Check sheet for the drawn part. Datum: minimum x, y, z corner. Units: mm. Give positions to 0.01 mm unless a question says otherwise; leave off trailing zeros. Order: outer loops, then holes, each group sorted by start corner. A loop starts at its lowest first (then second) coordinate and runs counter-clockwise, first axis right, second up. Notation, with made-up numbers: M 33.5,-34.5 L 64.5,-34.5 A34 cw 64.5,4.5 Z; hole C 55,84 d11. An arc over 180 degrees is marked long. Put each result on its own line as item: value. Start each with the question number.
Q1. Section check C-C on z = 6.5. Record the cut outline in (x, y), then the cut area to 3 significant figures.
Q2. Section check A-A on y = 13. Record the cut outline in (x, z), then the cut area to 3 significant figures.
Q3. Material ranges on L1, parallel to Y at x = 13, z = 4; L2, parallel to Y at x = 9, z = 7.25; L3, parallel to X at y = 10.5, z = 4.25, recorded low to high.
Q4. Mould release check, pull along Y, two halves, no side actions. Record for the marked faces 1, 2 and 3: +Y half, -Y half, draft (parallel to the pull), parting line (faces both ways), or undercut.
Q5. Go/stop test with flat-tipped pins: pin 1 (1 mm diameter, centred on x = 15.5, z = 4, fed in from -Y); pin 2 (2 mm diameter, centred on x = 9.5, z = 1.5, fed in from +Y); pin 3 (8 mm diameter, centred on x = 13, y = 13, fed in from -Z); pin 4 (4 mm diameter, centred on y = 21.5, z = 5.5, fed in from -X). Record where each tip stops, or that it passes through.
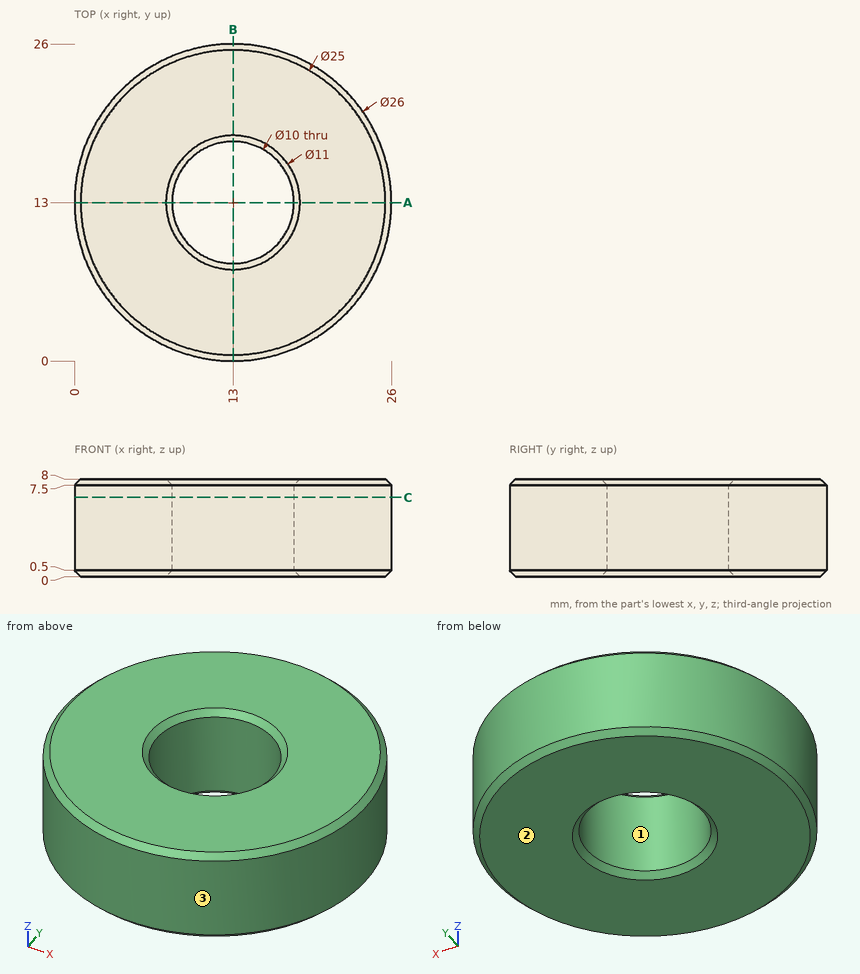
Results found:
1. outline: C 13,13 d26; hole C 13,13 d10
1. area: 452 mm^2
2. outline: M 0,0.5 L 0.5,0 L 7.5,0 L 8,0.5 L 8,7.5 L 7.5,8 L 0.5,8 L 0,7.5 Z; M 18,0.5 L 18.5,0 L 25.5,0 L 26,0.5 L 26,7.5 L 25.5,8 L 18.5,8 L 18,7.5 Z
2. area: 127 mm^2
3. L1: y = 0 to 8, 18 to 26
3. L2: y = 0.63 to 10, 16 to 25.37
3. L3: x = 0.24 to 8.67, 17.33 to 25.76
4. face 1: undercut
4. face 2: draft
4. face 3: parting line
5. pin 1: stops at y = 0.15
5. pin 2: stops at y = 25.76
5. pin 3: passes through
5. pin 4: stops at x = 1.74
